Autodesk Inventor part; units mm, degrees
ref_plane "YZ Plane" through (0, 0, 0) normal (1, 0, 0) x (0, 1, 0)
ref_plane "XZ Plane" through (0, 0, 0) normal (0, 1, 0) x (-1, 0, 0)
ref_plane "XY Plane" through (0, 0, 0) normal (0, 0, 1) x (1, 0, 0)
sketch "Sketch6" plane through (0, 0, 0) normal (0, 1, 0) x (-1, 0, 0)
  line L0 (450, -490) -> (-450, -490)
  line L1 (-450, -490) -> (-450, 490)
  line L2 (-450, 490) -> (450, 490)
  line L3 (450, 490) -> (450, -490)
  line L4 (450, -490) -> (-450, 490) construction
  line L5 (-450, -490) -> (450, 490) construction
  point P0 (0, 0)
  dimension "d52" = 900
  dimension "d53" = 980
extrude "Plate2" add sketch "Sketch6" along normal blind 0.5
sketch "Sketch11" plane through (449.5, 0, -490) normal (1, 0, 0) x (0, 1, 0)
  line L0 (0, 980) -> (0, 0)
  line L1 (0, 0) -> (10, 0)
  line L2 (10, 0) -> (10, 980)
  line L3 (10, 980) -> (0, 980)
edge flange "Flange2" height 10 angle 90 thickness 0.5 bend radius 0.5 thickness toward (1, 0, 0) relief tear relief width 0.5 relief depth 0.25 edges at (450, 0.5, 0) wall of the first edge with corners at (449.5, 0, 490) (449.5, 0, -490) (449.5, 10, -490) (449.5, 10, 490)
bend "Bend3"
corner "Corner3"
sketch "Sketch12" plane through (450, 9.5, -490) normal (0, 1, 0) x (-1, 0, 0)
  line L0 (0, 980) -> (0, 0)
  line L1 (0, 0) -> (10, 0)
  line L2 (10, 0) -> (10, 980)
  line L3 (10, 980) -> (0, 980)
edge flange "Flange3" height 10 angle 90 thickness 0.5 bend radius 0.5 thickness toward (0, 1, 0) relief tear relief width 0.5 relief depth 0.25 edges at (449.5, 10, 0) wall of the first edge with corners at (450, 9.5, 490) (450, 9.5, -490) (440, 9.5, -490) (440, 9.5, 490)
bend "Bend4"
corner "Corner4"
sketch "Sketch13" plane through (-449.5, 0, 490) normal (-1, 0, 0) x (0, -1, 0)
  line L0 (0, -980) -> (0, 0)
  line L1 (0, 0) -> (-10, 0)
  line L2 (-10, 0) -> (-10, -980)
  line L3 (-10, -980) -> (0, -980)
edge flange "Flange4" height 10 angle 90 thickness 0.5 bend radius 0.5 thickness toward (-1, 0, 0) relief tear relief width 0.5 relief depth 0.25 edges at (-450, 0.5, 0) wall of the first edge with corners at (-449.5, 0, -490) (-449.5, 0, 490) (-449.5, 10, 490) (-449.5, 10, -490)
bend "Bend5"
corner "Corner5"
sketch "Sketch14" plane through (-450, 9.5, 490) normal (0, 1, 0) x (-1, 0, 0)
  line L0 (0, -980) -> (0, 0)
  line L1 (0, 0) -> (-10, 0)
  line L2 (-10, 0) -> (-10, -980)
  line L3 (-10, -980) -> (0, -980)
edge flange "Flange5" height 10 angle 90 thickness 0.5 bend radius 0.5 thickness toward (0, 1, 0) relief tear relief width 0.5 relief depth 0.25 edges at (-449.5, 10, 0) wall of the first edge with corners at (-450, 9.5, -490) (-450, 9.5, 490) (-440, 9.5, 490) (-440, 9.5, -490)
bend "Bend6"
corner "Corner6"
equation "\"d52\" = ЖАБРЫ_базовая_ширина - ЖАБРЫ_коррекция"
equation "\"d53\" = ЖАБРЫ_базовая_длина_кор_лист"
equation "\"d54\" = Thickness"
equation "\"d84\" = BendReliefWidth"
equation "\"d85\" = BendReliefDepth"
equation "\"d86\" = MinimumRemnant"
equation "\"d87\" = TransitionRadius"
equation "\"d90\" = BendRadius"
equation "\"d91\" = CornerReliefSize"
equation "\"d92\" = GapSize"
equation "\"d93\" = JacobiRadiusSize"
equation "\"d94\" = BendReliefWidth"
equation "\"d95\" = BendReliefDepth"
equation "\"d96\" = MinimumRemnant"
equation "\"d97\" = TransitionRadius"
equation "\"d100\" = BendRadius"
equation "\"d101\" = CornerReliefSize"
equation "\"d102\" = GapSize"
equation "\"d103\" = JacobiRadiusSize"
equation "\"d104\" = BendReliefWidth"
equation "\"d105\" = BendReliefDepth"
equation "\"d106\" = MinimumRemnant"
equation "\"d107\" = TransitionRadius"
equation "\"d110\" = BendRadius"
equation "\"d111\" = CornerReliefSize"
equation "\"d112\" = GapSize"
equation "\"d113\" = JacobiRadiusSize"
equation "\"d114\" = BendReliefWidth"
equation "\"d115\" = BendReliefDepth"
equation "\"d116\" = MinimumRemnant"
equation "\"d117\" = TransitionRadius"
equation "\"d120\" = BendRadius"
equation "\"d121\" = CornerReliefSize"
equation "\"d122\" = GapSize"
equation "\"d123\" = JacobiRadiusSize"
equation "\"BendRadius\" = Thickness"
equation "\"BendReliefWidth\" = Thickness"
equation "\"BendReliefDepth\" = 0.5 * Thickness"
equation "\"CornerReliefSize\" = 4 * Thickness"
equation "\"MinimumRemnant\" = 2 * Thickness"
equation "\"TransitionRadius\" = BendRadius"
equation "\"JacobiRadiusSize\" = BendRadius"
equation "\"GapSize\" = Thickness"
properties part number "MSC 803 sheet gills" material "Stainless Steel"
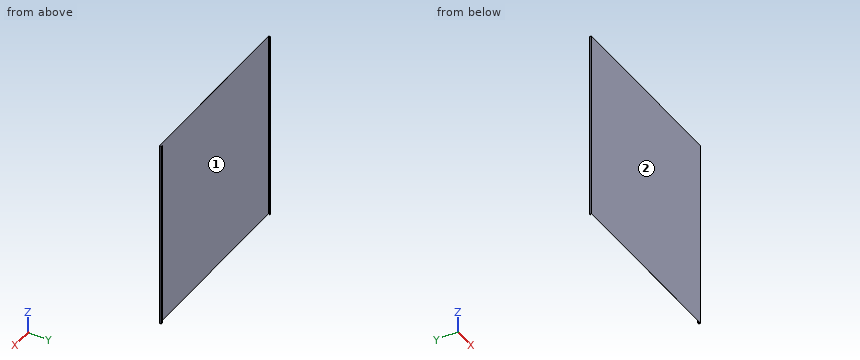
Design review of the part built by this model. Coordinates are the model's own, in mm. Face numbers are marked on the shaded views. Coordinates: 2 decimals unless noted, no trailing zeros. Write each loop counter-clockwise with the first axis right and the second up, starting at its lowest first coordinate (ties: lowest second). Pieces come first, ordered by that corner, then holes. Notation, with made-up numbers: M -11.5,62.25 L 46.5,62.25 A33 ccw 46.5,97.25 Z; hole C -25,42 d10. An arc over 180 degrees is marked long. Answer as a JSON object with one key per item and string values.
Item 1: Draft analysis for pull direction X (two halves, no side actions). For the marked faces 1 and 2, state which applies: pulls with the +X half, pulls with the -X half, needs draft (parallel to the pull), parting line crosses it, or undercut.
Outcome:
{"face 1": "undercut", "face 2": "needs draft"}
Item 2: Wall thickness on probe 1 along X at (y, z) = (4.75, -53); probe 2 along Y at (x, z) = (-18, -83.5): over which ranges is each line inside the solid? List them lowest first.
Outcome:
{"probe 1": "-450 to -449.5, 449.5 to 450", "probe 2": "0 to 0.5"}
Item 3: Add section C-C, the plane x = 237.5. Give the boundary of the cut face in (y, z), and give its area (3 significant figures).
Outcome:
{"outline": "M 0,-490 L 0.5,-490 L 0.5,490 L 0,490 Z", "area": "490 mm²"}
Item 4: Add section A-A, the plane y = 5.75. Give the boundary of the cut face in (x, z).
Outcome:
{"outline": "M -450,-490 L -449.5,-490 L -449.5,490 L -450,490 Z; M 449.5,-490 L 450,-490 L 450,490 L 449.5,490 Z"}
Item 5: Insertion check: pin 1 Ø4 at (x, z) = (125.5, 151.5) entering from +Y. The pin has a flat end and moves straight along its axis. Give the tip position at first contact, or say it passes through.
Outcome:
{"pin 1": "y = 0.5"}
Item 6: Add section B-B, the plane z = -403.5. Give the boundary of the cut face in (x, y), and give its area (3 significant figures).
Outcome:
{"outline": "M -450,1 A1 ccw -449,0 L 449,0 A1 ccw 450,1 L 450,9 A1 ccw 449,10 L 440,10 L 440,9.5 L 449,9.5 A0.5 cw 449.5,9 L 449.5,1 A0.5 cw 449,0.5 L -449,0.5 A0.5 cw -449.5,1 L -449.5,9 A0.5 cw -449,9.5 L -440,9.5 L -440,10 L -449,10 A1 ccw -450,9 Z", "area": "468 mm²"}
